```python
from build123d import *

# Parameters (mm, degrees)
F0_W     = 114.7212088108
F0_H     = 84.7007036209
F1_DEPTH = 152.4
F2_W     = 4.020601511
F2_H     = 68.6182938516
F3_DEPTH = 152.4
F4_T     = -2.54
F5_DEPTH = 152.401
F6_DEPTH = 152.401
F7_DEPTH = 152.401
F8_DEPTH = 152.401


with BuildPart() as f1:
    # F0 (on Front) → F1 (new body)
    with BuildSketch(Plane.XZ):
        with Locations((1.1391714215, 1.8092729151)):
            Rectangle(F0_W, F0_H)
    extrude(amount=F1_DEPTH)

    # F2 (on face) → F3 (cut)
    with BuildSketch(Plane.XZ.offset(152.4)):
        with Locations((-46.1699254811, -0.3350507468)):
            Rectangle(F2_W, F2_H)
    extrude(amount=-F3_DEPTH, mode=Mode.SUBTRACT)

    # F4
    f4_openings = [f1.faces().sort_by_distance(p)[0] for p in [
        (-56.221433, -76.2, 1.809273),
        (58.499776, -76.2, 1.809273),
    ]]
    offset(amount=F4_T, openings=f4_openings, kind=Kind.INTERSECTION)

    # F2 (on face) → F5 (cut, through all)
    with BuildSketch(Plane.XZ.offset(152.4)):
        Rectangle(F2_W, F2_H)
    extrude(amount=-F5_DEPTH, mode=Mode.SUBTRACT)

    # F2 (on face) → F6 (cut, through all)
    with BuildSketch(Plane.XZ.offset(152.4)):
        with Locations((-23.0849627405, -0.1675253734)):
            Rectangle(F2_W, F2_H)
        with Locations((23.0849627405, 0.1675253734)):
            Rectangle(F2_W, F2_H)
    extrude(amount=-F6_DEPTH, mode=Mode.SUBTRACT)

    # F2 (on face) → F7 (cut, through all)
    with BuildSketch(Plane.XZ.offset(152.4)):
        with Locations((-34.6274441108, -0.2512880601)):
            Rectangle(F2_W, F2_H)
        with Locations((-11.5424813703, -0.0837626867)):
            Rectangle(F2_W, F2_H)
        with Locations((11.5424813703, 0.0837626867)):
            Rectangle(F2_W, F2_H)
        with Locations((34.6274441108, 0.2512880601)):
            Rectangle(F2_W, F2_H)
    extrude(amount=-F7_DEPTH, mode=Mode.SUBTRACT)

    # F2 (on face) → F8 (cut, through all)
    with BuildSketch(Plane.XZ.offset(152.4)):
        with Locations((-40.3986847959, -0.2931694034)):
            Rectangle(F2_W, F2_H)
        with Locations((-28.8562034257, -0.2094067167)):
            Rectangle(F2_W, F2_H)
        with Locations((-17.3137220554, -0.12564403)):
            Rectangle(F2_W, F2_H)
        with Locations((-5.7712406851, -0.0418813433)):
            Rectangle(F2_W, F2_H)
        with Locations((5.7712406851, 0.0418813433)):
            Rectangle(F2_W, F2_H)
        with Locations((17.3137220554, 0.12564403)):
            Rectangle(F2_W, F2_H)
        with Locations((28.8562034257, 0.2094067167)):
            Rectangle(F2_W, F2_H)
        with Locations((40.3986847959, 0.2931694034)):
            Rectangle(F2_W, F2_H)
    extrude(amount=-F8_DEPTH, mode=Mode.SUBTRACT)


solid = f1.part
```
The model under review builds one solid part; all positions refer to its coordinate system, in mm. A direction names the side the tool comes from. Round coordinates to 2 decimals unless told otherwise and drop trailing zeros. Loops run counter-clockwise (first coordinate to the right, second up) from the corner with the lowest first, then second, coordinate; pieces in that order, holes last.
Item 1: For faces 1 (the face through (-42, -88, 34.016)), 2 (the face through (-46, -77, -37.184)), 3 (the face through (-56.221, -53, 42)), list the 3-axis set-ups (+Z, -Z, +X, -X, +Y, -Y) from which the entire face can be reached by the end or side of a thin tool; tool diameter is ignored.
Determined:
face 1: +Y, -Y
face 2: +X, -X
face 3: +Z, -Z, -X, +Y, -Y
Item 2: Mouldability with a two-part tool opening along Y and no side actions: class faces 4 (the face through (26, -2.54, 2)), 5 (the face through (-50.72, -77, -1)), 6 (the face through (-42, -88, -34.602)), 7 (the face through (26, -152.4, 2)) as released by +Y, released by -Y, zero draft, split by the parting line, or undercut.
Determined:
face 4: undercut
face 5: undercut
face 6: zero draft
face 7: released by -Y
Item 3: Take a section at C-C (z = -16). Give the number of separate pieces and of enclosed holes in the cut face, then the cut area to 3 significant figures.
Determined:
separate pieces: 32
enclosed holes: 0
area: 888 mm2
Item 4: Take a section at B-B (x = -17.5). Write out the cut boundary in (y, z), then the cut area to 3 significant figures.
Determined:
outline: (-152.4, -40.54) - (0, -40.54) - (0, -34.43) - (-2.54, -34.43) - (-2.54, -38) - (-149.86, -38) - (-149.86, -34.43) - (-152.4, -34.43) - close; (-152.4, 34.18) - (-149.86, 34.18) - (-149.86, 41.62) - (-2.54, 41.62) - (-2.54, 34.18) - (0, 34.18) - (0, 44.16) - (-152.4, 44.16) - close
area: 830 mm2
Item 5: Clearance check with flat-ended pins moving along their axes: pin 1 Ø1.2 at (y, z) = (-88.5, 36) entering from +X; pin 2 Ø1.5 at (y, z) = (-35, -1) entering from +X; pin 3 Ø1.5 at (y, z) = (-96, 23.5) entering from -X. State where each tip first meets the part, or that it passes through.
Determined:
pin 1: stops at x = -41.62
pin 2: stops at x = -42.41
pin 3: stops at x = -50.72
Item 6: For line 1 (Z direction, x = 42, y = -91); line 2 (X direction, y = -105, z = -25.5); line 3 (Y direction, x = 40.5, z = 40), list the stretches that pass through material, from the lowest coordinate up.
Determined:
line 1: z = -40.54 to -38, 41.62 to 44.16
line 2: x = -50.72 to -48.18, -44.16 to -42.41
line 3: y = -152.4 to -149.86, -2.54 to 0
Item 7: Take a section at A-A (y = -118). Write out the cut boundary in (x, z).
Determined:
outline: (-56.22, -40.54) - (58.5, -40.54) - (58.5, -38) - (-56.22, -38) - close; (-56.22, 41.62) - (58.5, 41.62) - (58.5, 44.16) - (-56.22, 44.16) - close; (-50.72, -37.18) - (-41.62, -37.18) - (-41.62, -34.6) - (-42.41, -34.6) - (-42.41, 34.02) - (-41.62, 34.02) - (-41.62, 36.51) - (-50.72, 36.51) - close; hole (-48.18, -34.64) - (-44.16, -34.64) - (-44.16, 33.97) - (-48.18, 33.97) - close
